from build123d import *

# Parameters (mm, degrees)
SKETCH1_W           = 40
SKETCH1_H           = 40
BOSS_EXTRUDE1_DEPTH = 260
SKETCH3_W           = 40
SKETCH3_H           = 40
SKETCH3_W_2         = 20
SKETCH3_H_2         = 20
CUT_EXTRUDE1_DEPTH  = 180
SKETCH4_W           = 30
SKETCH4_H           = 30
CUT_EXTRUDE2_DEPTH  = 264.818119165


with BuildPart() as part:
    # Sketch1 → Boss-Extrude1 (new body)
    with BuildSketch(Plane.XY):
        Rectangle(SKETCH1_W, SKETCH1_H)
    extrude(amount=BOSS_EXTRUDE1_DEPTH)

    # Sketch3 → Cut-Extrude1 (cut)
    with BuildSketch(Plane.XY.offset(220)):
        Rectangle(SKETCH3_W, SKETCH3_H)
        Rectangle(SKETCH3_W_2, SKETCH3_H_2, mode=Mode.SUBTRACT)
    extrude(amount=-CUT_EXTRUDE1_DEPTH, mode=Mode.SUBTRACT)

    # Sketch4 → Cut-Extrude2 (cut, through all)
    with BuildSketch(Plane.ZY.offset(20)):
        with Locations((20, 0)):
            Rectangle(SKETCH4_W, SKETCH4_H)
        with Locations((240, 0)):
            Rectangle(SKETCH4_W, SKETCH4_H)
    extrude(amount=-CUT_EXTRUDE2_DEPTH, mode=Mode.SUBTRACT)


solid = part.part
Part model, mm, in its own coordinate system. A direction names the side the tool comes from. Coordinates: 2 decimals unless noted, no trailing zeros. Write each loop counter-clockwise with the first axis right and the second up, starting at its lowest first coordinate (ties: lowest second). Pieces come first, ordered by that corner, then holes. Notation, with made-up numbers: (-14, 70.25) - (-3, 70.25) arc R26 cw to (-3, 86.25) - close; hole circle Ø7 at (-3, 41.5). An arc over 180 degrees is marked (long way). Put each result on its own line as item: value.
1. Flat gauge pins, fed straight in: pin 1 Ø6 at (y, z) = (2, 111.5) entering from -X; pin 2 Ø2 at (x, z) = (9.5, 91) entering from +Y; pin 3 Ø22 at (y, z) = (1, 108.5) entering from +X. Where does each tip first touch, or does it go through?
Final values:
pin 1: stops at x = -10
pin 2: stops at y = 10
pin 3: stops at x = 10
2. Probe line 1 along Z through (x, y) = (7, 9.5); line 2 along Z through (x, y) = (-4, -14.5); line 3 along Y through (x, z) = (2.5, 168). List the from-to ranges inside material, lowest first. Write a range as [from, to].
Final values:
line 1: z = [0, 5], [35, 225], [255, 260]
line 2: z = [0, 5], [35, 40], [220, 225], [255, 260]
line 3: y = [-10, 10]
3. Band-saw the part on B-B (x = 16.5). Write the cut outline in (y, z), then the cut area to 3 significant figures.
Final values:
outline: (-20, 0) - (20, 0) - (20, 40) - (-20, 40) - close; (-20, 220) - (20, 220) - (20, 260) - (-20, 260) - close; hole (-15, 5) - (15, 5) - (15, 35) - (-15, 35) - close; hole (-15, 225) - (15, 225) - (15, 255) - (-15, 255) - close
area: 1,400 mm²
4. Band-saw the part on C-C (z = 43.5). Write the cut outline in (x, y), then the cut area to 3 significant figures.
Final values:
outline: (-10, -10) - (10, -10) - (10, 10) - (-10, 10) - close
area: 400 mm²
5. Band-saw the part on A-A (y = 3). Write the cut outline in (x, z), then the cut area to 3 significant figures.
Final values:
outline: (-20, 0) - (20, 0) - (20, 5) - (-20, 5) - close; (-20, 35) - (20, 35) - (20, 40) - (10, 40) - (10, 220) - (20, 220) - (20, 225) - (-20, 225) - (-20, 220) - (-10, 220) - (-10, 40) - (-20, 40) - close; (-20, 255) - (20, 255) - (20, 260) - (-20, 260) - close
area: 4,400 mm²
6. 3-axis set-ups, long thin cutter, end or side, ignore diameter. For faces 1 (the flat face through (0, 0, 5)), 2 (the flat face through (0, 14, 220)), 3 (the flat face through (0, 10, 131)): which of +Z, -Z, +X, -X, +Y, -Y reach the whole face in a straight line?
Final values:
face 1: +X, -X
face 2: none
face 3: +X, -X, +Y
7. Two-plate mould, pull along Z, no slides. Class faces 4 (the flat face through (0, 20, 20)), 5 (the flat face through (0, -15, 240)), 6 (the flat face through (0, 0, 0)): +Z half, -Z half, draft (parallel to the pull), parting line (faces both ways), or undercut.
Final values:
face 4: draft
face 5: undercut
face 6: -Z half
